Print and shaded views of the part. All mm, measured from the part's lowest x, y and z. Round coordinates to 2 decimals unless told otherwise and drop trailing zeros. Write each loop counter-clockwise with the first axis right and the second up, starting at its lowest first coordinate (ties: lowest second). Pieces come first, ordered by that corner, then holes. Notation, with made-up numbers: (31.25, 85) - (38.25, 85) arc R27 cw to (38.25, 112) - close; hole circle Ø6 at (48, -38.5). An arc over 180 degrees is marked (long way). Put each result on its own line as item: value. Start each with the question number.
Item 1: Cut at B-B (x = 82.5). Give the cut face in (y, z) (3 decimals).
Item 2: Cut at A-A (z = 5). Give the cut face in (x, y).
Item 3: Drill centre lines: line 1 (Y direction, x = 44, z = 6); line 2 (X direction, y = 49.5, z = 3.75); line 3 (Z direction, x = 70, y = 188.5). Where is each one in solid material? Low to high. Write a range as from..to.
Item 4: Mould opens along Y. For the marked faces 1 and 2 say: released by +Y, released by -Y, zero draft, split by the parting line, or undercut.
Item 5: Cut at C-C (y = 81.5). Give the cut face in (x, z) (3 decimals), and give its area (3 significant figures).
Item 6: Pin check, flat tips, straight feed: pin 1 Ø1 at (x, z) = (81, 5.5) entering from +Y; pin 2 Ø1.9 at (x, z) = (62.5, 4) entering from -Y; pin 3 Ø3 at (y, z) = (48.5, 4.5) entering from -X. Stop position of each tip, or through.
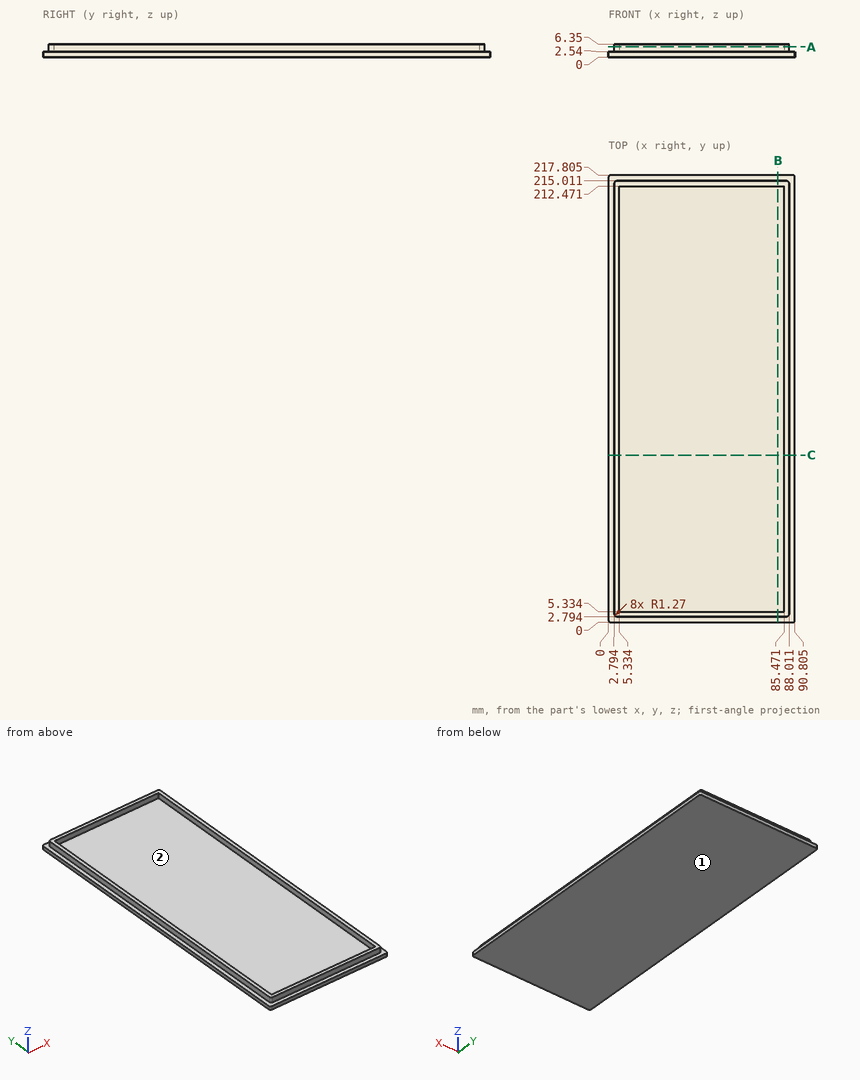
Output values:
1. outline: (0, 0) - (217.805, 0) - (217.805, 2.54) - (215.011, 2.54) - (215.011, 6.35) - (212.471, 6.35) - (212.471, 2.54) - (5.334, 2.54) - (5.334, 6.35) - (2.794, 6.35) - (2.794, 2.54) - (0, 2.54) - close
2. outline: (2.79, 4.06) arc R1.27 ccw to (4.06, 2.79) - (86.74, 2.79) arc R1.27 ccw to (88.01, 4.06) - (88.01, 213.74) arc R1.27 ccw to (86.74, 215.01) - (4.06, 215.01) arc R1.27 ccw to (2.79, 213.74) - close; hole (5.33, 5.33) - (85.47, 5.33) - (85.47, 212.47) - (5.33, 212.47) - close
3. line 1: 2.79..5.33, 212.47..215.01
3. line 2: 2.79..5.33, 85.47..88.01
3. line 3: 0..2.54
4. face 1: zero draft
4. face 2: undercut
5. outline: (0, 0) - (90.805, 0) - (90.805, 2.54) - (88.011, 2.54) - (88.011, 6.35) - (85.471, 6.35) - (85.471, 2.54) - (5.334, 2.54) - (5.334, 6.35) - (2.794, 6.35) - (2.794, 2.54) - (0, 2.54) - close
5. area: 250 mm2
6. pin 1: y = 215.01
6. pin 2: y = 2.79
6. pin 3: x = 2.79
